```python
from build123d import *

# Parameters (mm, degrees)
SKETCH1_W                = 90
SKETCH1_H                = 90
BOSS_EXTRUDE1_DEPTH      = 1.25
M4_CLEARANCE_HOLE1_D     = 4.5
M4_CLEARANCE_HOLE1_DEPTH = 5.2
M4_CLEARANCE_HOLE1_TIP   = 1.351936393


with BuildPart() as part:
    # Sketch1 → Boss-Extrude1 (new, symmetric)
    with BuildSketch(Plane(origin=(0, 0, 0), x_dir=(1, 0, 0), z_dir=(0, 1, 0))):
        Rectangle(SKETCH1_W, SKETCH1_H)
    extrude(amount=BOSS_EXTRUDE1_DEPTH, both=True)

    # M4 Clearance Hole1
    with Locations(Plane(origin=(0, 1.25, 0), x_dir=(1, 0, 0), z_dir=(0, 1, 0))):
        with Locations((0, 0), (15.25, 15.25), (-15.25, -15.25), (-15.25, 15.25), (15.25, -15.25)):
            Hole(M4_CLEARANCE_HOLE1_D / 2, depth=M4_CLEARANCE_HOLE1_DEPTH)
            with Locations((0, 0, -(M4_CLEARANCE_HOLE1_DEPTH + M4_CLEARANCE_HOLE1_TIP / 2))):  # 118° drill point
                Cone(0, M4_CLEARANCE_HOLE1_D / 2, M4_CLEARANCE_HOLE1_TIP, mode=Mode.SUBTRACT)


solid = part.part
```
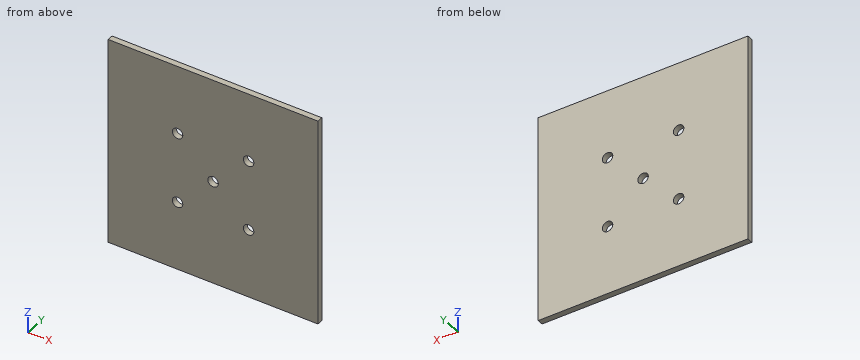
Design review of the part built by this model. Coordinates are the model's own, in mm. Coordinates: 2 decimals unless noted, no trailing zeros. Order: outer loops, then holes, each group sorted by start corner. A loop starts at its lowest first (then second) coordinate and runs counter-clockwise, first axis right, second up.
1) Wall thickness on line 1 along X through (y, z) = (0.7, -15.25); line 2 along Z through (x, y) = (13.5, 1.05): over which ranges is each line inside the solid? List them lowest first.
2) Take a section at A-A, the plane z = 0. Give the boundary of the cut face in (x, y).
3) Take a section at B-B, the plane x = -15.25. Give the boundary of the cut face in (y, z), and give its area (4 significant figures).
4) Clearance check with a flat-ended pin moving along its axis: pin 1 (3.5 mm diameter, centred on x = 15.25, z = 15.25, fed in from -Y). State where the tip first meets the part, or that it passes through.
5) Take a section at C-C, the plane x = 0. Give the boundary of the cut face in (y, z).
Returned:
1. line 1: x = -45 to -17.5, -13 to 13, 17.5 to 45
1. line 2: z = -45 to -16.66, -13.84 to 13.84, 16.66 to 45
2. outline: (-45, -1.25) - (-2.25, -1.25) - (-2.25, 1.25) - (-45, 1.25) - close; (2.25, -1.25) - (45, -1.25) - (45, 1.25) - (2.25, 1.25) - close
3. outline: (-1.25, -45) - (1.25, -45) - (1.25, -17.5) - (-1.25, -17.5) - close; (-1.25, -13) - (1.25, -13) - (1.25, 13) - (-1.25, 13) - close; (-1.25, 17.5) - (1.25, 17.5) - (1.25, 45) - (-1.25, 45) - close
3. area: 202.5 mm2
4. pin 1: passes through
5. outline: (-1.25, -45) - (1.25, -45) - (1.25, -2.25) - (-1.25, -2.25) - close; (-1.25, 2.25) - (1.25, 2.25) - (1.25, 45) - (-1.25, 45) - close
